Geometry check sheet. Reference: drawing and pictorial views, mm from the part's lowest x, y, z. Coordinates: 2 decimals unless noted, no trailing zeros. Loops run counter-clockwise (first coordinate to the right, second up) from the corner with the lowest first, then second, coordinate; pieces in that order, holes last. Notation, with made-up numbers: (-34, -5) -> (23, -5) arc R11 ccw to (23, 4) -> close; hole circle Ø9 at (35, 28.5). An arc over 180 degrees is marked (long way). Answer as a JSON object with one key per item and string values. Group by question number.
Q1. Cross-section at C-C on x = 10. Record the boundary of the cut face in (y, z), and give its area (3 significant figures).
Q2. Gauge pin test, flat ends, axial feed: pin 1 Ø1 at (x, y) = (9, 3) entering from +Z; pin 2 Ø1.5 at (x, z) = (10.5, 1) entering from +Y. Record the tip position at first contact, or that the pin passes through.
Q3. Release check for a two-part mould opening along X. For the marked faces 1, 2, 3 and 4 record: released by +X, released by -X, zero draft, split by the parting line, or undercut.
Q4. Scan lines: L1, parallel to Y at x = 10.5, z = 1.9; L2, parallel to X at y = 2.6, z = 3; L3, parallel to X at y = 2.2, z = 1.1. Record each from-to range of solid material in increasing order.
Q5. Cross-section at B-B on y = 2. Record the boundary of the cut face in (x, z).
Q6. Cross-section at A-A on z = 2. Record the boundary of the cut face in (x, y).
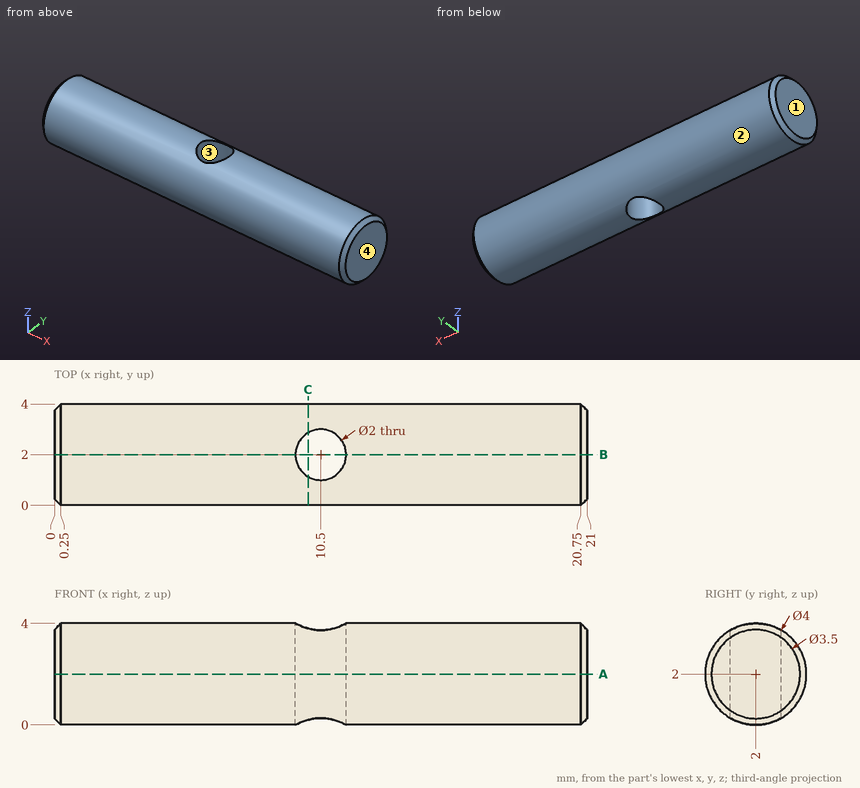
Computed values:
{
 "1": {"outline": "(1.13, 0.2) -> (1.13, 3.8) arc R2 ccw to start; (2.87, 0.2) arc R2 ccw to (2.87, 3.8) -> close", "area": "5.86 mm²"},
 "2": {"pin 1": "stops at z = 3.94", "pin 2": "stops at y = 3.98"},
 "3": {"face 1": "released by -X", "face 2": "zero draft", "face 3": "undercut", "face 4": "released by +X"},
 "4": {"L1": "y = 0 to 1, 3 to 4", "L2": "x = 0 to 9.7, 11.3 to 21", "L3": "x = 0 to 9.52, 11.48 to 21"},
 "5": {"outline": "(0, 0.25) -> (0.25, 0) -> (9.5, 0) -> (9.5, 4) -> (0.25, 4) -> (0, 3.75) -> close; (11.5, 0) -> (20.75, 0) -> (21, 0.25) -> (21, 3.75) -> (20.75, 4) -> (11.5, 4) -> close"},
 "6": {"outline": "(0, 0.25) -> (0.25, 0) -> (20.75, 0) -> (21, 0.25) -> (21, 3.75) -> (20.75, 4) -> (0.25, 4) -> (0, 3.75) -> close; hole circle Ø2 at (10.5, 2)"}
}
